```python
from build123d import *

# Parameters (mm, degrees)
SKETCH1_R           = 1.25
BOSS_EXTRUDE1_DEPTH = 1
BOSS_EXTRUDE2_START = 5
BOSS_EXTRUDE2_DEPTH = 5


with BuildPart() as part:
    # Sketch1 → Boss-Extrude1 (new body)
    with BuildSketch(Plane.XY):
        with BuildLine():
            Line((10.812920647, 4.222556691), (7.37, 2.234785529))
            ThreePointArc((7.37, 2.234785529), (4.979455543, 2.875329985), (5.62, 5.265874442))
            Line((5.62, 5.265874442), (6.546167381, 5.800597429))
            ThreePointArc((6.546167381, 5.800597429), (7.040499888, 6.560307898), (6.717963757, 7.407358703))
            ThreePointArc((6.717963757, 7.407358703), (0, 10), (-6.717963757, 7.407358703))
            ThreePointArc((-6.717963757, 7.407358703), (-7.040499888, 6.560307898), (-6.546167381, 5.800597429))
            Line((-6.546167381, 5.800597429), (-5.62, 5.265874442))
            ThreePointArc((-5.62, 5.265874442), (-4.979455543, 2.875329985), (-7.37, 2.234785529))
            Line((-7.37, 2.234785529), (-10.812920647, 4.222556691))
            ThreePointArc((-10.812920647, 4.222556691), (-11.269892812, 4.798402367), (-11.209696355, 5.531067494))
            ThreePointArc((-11.209696355, 5.531067494), (0, 12.5), (11.209696355, 5.531067494))
            ThreePointArc((11.209696355, 5.531067494), (11.269892812, 4.798402367), (10.812920647, 4.222556691))
        make_face()
        with Locations((-6.495, 3.750329985)):
            Circle(SKETCH1_R, mode=Mode.SUBTRACT)
        with Locations((6.495, 3.750329985)):
            Circle(SKETCH1_R, mode=Mode.SUBTRACT)
    extrude(amount=-BOSS_EXTRUDE1_DEPTH)

    # Sketch2 → Boss-Extrude2 (add)
    with BuildSketch(Plane.XY.offset(BOSS_EXTRUDE2_START)):
        with BuildLine():
            Line((9.361858429, 3.384785529), (8.486858429, 4.900329985))
            Line((8.486858429, 4.900329985), (10, 7.5))
            ThreePointArc((10, 7.5), (10.650444999, 6.543548069), (11.209696355, 5.531067494))
            ThreePointArc((11.209696355, 5.531067494), (11.269892812, 4.798402367), (10.812920647, 4.222556691))
            Line((10.812920647, 4.222556691), (9.361858429, 3.384785529))
        make_face()
        with BuildLine():
            Line((-9.361858429, 3.384785529), (-10.812920647, 4.222556691))
            ThreePointArc((-10.812920647, 4.222556691), (-11.269892812, 4.798402367), (-11.209696355, 5.531067494))
            ThreePointArc((-11.209696355, 5.531067494), (-10.650444999, 6.543548069), (-10, 7.5))
            Line((-10, 7.5), (-8.486858429, 4.900329985))
            Line((-8.486858429, 4.900329985), (-9.361858429, 3.384785529))
        make_face()
    extrude(amount=-BOSS_EXTRUDE2_DEPTH)


solid = part.part
```
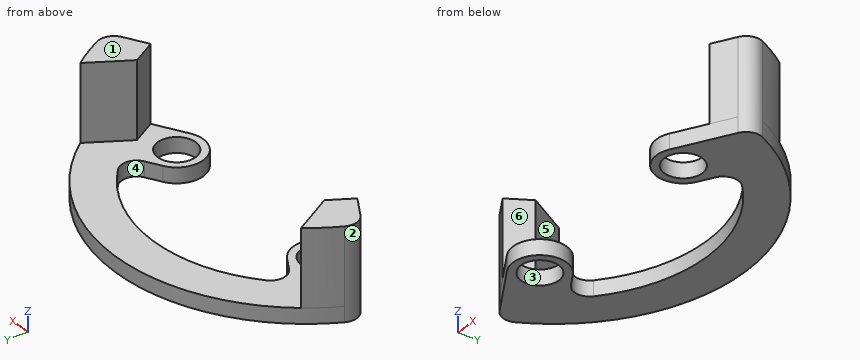
For this review, take the finished solid that the model builds, in its own axes (mm). Face numbers are marked on the shaded views. A direction names the side the tool comes from. Coordinates: 2 decimals unless noted, no trailing zeros. Loops run counter-clockwise (first coordinate to the right, second up) from the corner with the lowest first, then second, coordinate; pieces in that order, holes last.
1. Add section B-B, the plane y = 7.75. Give the boundary of the cut face in (x, z), then the cut area to 3 significant figures.
2. Add section C-C, the plane x = 9.75. Give the boundary of the cut face in (y, z).
3. Add section A-A, the plane z = 1.8. Give the boundary of the cut face in (x, y).
4. For line 1 (X direction, y = 3, z = -0.3); line 2 (Z direction, x = 4.5, y = 9.5); line 3 (X direction, y = 4, z = 2.1), list the stretches that pass through material, from the lowest coordinate up.
5. Insertion check: P1, Ø3, axis at x = -3.5, y = 6, coming from the +Z side; P2, Ø3, axis at x = -6.5, y = 3.75, coming from the +Z side; P3, Ø1, axis at x = -8.5, z = 2, coming from the +Y side. Each pin has a flat end and moves straight along its axis. Give the tip position at first contact, or say it passes through.
6. Mouldability with a two-part tool opening along X and no side actions: class the marked faces 1, 2 and 3 as +X half, -X half, draft (parallel to the pull), parting line (faces both ways), or undercut.
7. Add section D-D, the plane y = 9. Give the boundary of the cut face in (x, z), then the cut area to 3 significant figures.
8. For the marked faces 4, 5 and 6, list the 3-axis set-ups (+Z, -Z, +X, -X, +Y, -Y) from which the entire face can be reached by the end or side of a thin tool; tool diameter is ignored.
Result:
1. outline: (-9.81, -1) - (-6.32, -1) - (-6.32, 0) - (-9.81, 0) - close; (6.32, -1) - (9.81, -1) - (9.81, 0) - (6.32, 0) - close
1. area: 6.98 mm2
2. outline: (3.61, -1) - (7.82, -1) - (7.82, 0) - (7.07, 0) - (7.07, 5) - (3.61, 5) - close
3. outline: (-11.21, 5.53) arc R1 ccw to (-10.81, 4.22) - (-9.36, 3.38) - (-8.49, 4.9) - (-10, 7.5) arc R12.5 ccw to start; (8.49, 4.9) - (9.36, 3.38) - (10.81, 4.22) arc R1 ccw to (11.21, 5.53) arc R12.5 ccw to (10, 7.5) - close
4. line 1: x = -8.7 to -7.49, -5.5 to -4.91, 4.91 to 5.5, 7.49 to 8.7
4. line 2: z = -1 to 0
4. line 3: x = -10.43 to -9.01, 9.01 to 10.43
5. P1: passes through
5. P2: stops at z = 0
5. P3: stops at y = 5.78
6. face 1: draft
6. face 2: -X half
6. face 3: undercut
7. outline: (-8.67, -1) - (-4.36, -1) - (-4.36, 0) - (-8.67, 0) - close; (4.36, -1) - (8.67, -1) - (8.67, 0) - (4.36, 0) - close
7. area: 8.63 mm2
8. face 4: +Z, -Z
8. face 5: +Z, +Y
8. face 6: +Z, -Y
